from build123d import *

# Parameters (mm, degrees)
SKETCH_1_W               = 3.76
SKETCH_1_H               = 11.54
SKETCH_1_W_2             = 1.83
SKETCH_1_W_3             = 14.6
SKETCH_1_H_2             = 2.72
SKETCH_1_H_3             = 6.9
EXTRUDE_1_DEPTH          = 1
SKETCH_1_3_W             = 3.76
SKETCH_1_3_H             = 11.54
SKETCH_1_3_W_2           = 1.83
SKETCH_1_3_W_3           = 14.6
SKETCH_1_3_H_2           = 2.72
EXTRUDE_2_DEPTH          = 10
EXTRUDE_3_DEPTH          = 14.6
CUT_EXTRUDE_1_DEPTH      = 14.6
CUT_EXTRUDE_2_DEPTH      = 14.6
CUT_EXTRUDE_3_DEPTH      = 14.6
PATTERN_CIRCULAR_1_COUNT = 2
SKETCH_7_W               = 20.64829466
SKETCH_7_H               = 2.860597992
CUT_EXTRUDE_4_DEPTH      = 38.6
SKETCH_8_W               = 54.18
SKETCH_8_H               = 19.048575036
SKETCH_8_W_2             = 7
SKETCH_8_H_2             = 4.5
SKETCH_8_R               = 1.6
EXTRUDE_4_DEPTH          = 1.5
SKETCH_9_W               = 54.18
SKETCH_9_H               = 1.8
EXTRUDE_5_DEPTH          = 7
SKETCH_10_R              = 1.65
CUT_EXTRUDE_5_DEPTH      = 5
EXTRUDE_START            = 2
SKETCH_8_3_W             = 7
SKETCH_8_3_H             = 4.5
SKETCH_8_3_R             = 1.6
EXTRUDE_6_DEPTH          = 2
SKETCH_11_W              = 54.18
SKETCH_11_H              = 6.653379434
CUT_EXTRUDE_6_DEPTH      = 5
CUT_EXTRUDE_7_DEPTH      = 54.18
SKETCH_13_W              = 8.99
SKETCH_13_H              = 1
EXTRUDE_7_DEPTH          = 10


with BuildPart() as part:
    # Sketch 1 → Extrude 1 (new body)
    # profile 1 of 6: a face of its own
    with BuildSketch(Plane(origin=(0, 0, 0), x_dir=(1, 0, 0), z_dir=(0, 1, 0))):
        Polygon((-7.603, 6.17), (-7.603, -6.17), (1.387, -6.17), (1.387, -3.45), (1.387, 3.45), (1.387, 6.17), align=None)
        with Locations((-4.723, 0)):
            Rectangle(SKETCH_1_W, SKETCH_1_H, mode=Mode.SUBTRACT)
        with Locations((-0.728, 0)):
            Rectangle(SKETCH_1_W_2, SKETCH_1_H, mode=Mode.SUBTRACT)
    # profile 2 of 6: a face of its own
    with BuildSketch(Plane(origin=(0, 0, 0), x_dir=(1, 0, 0), z_dir=(0, 1, 0))):
        with Locations((8.687, -4.81)):
            Rectangle(SKETCH_1_W_3, SKETCH_1_H_2)
    # profile 3 of 6: a face of its own
    with BuildSketch(Plane(origin=(0, 0, 0), x_dir=(1, 0, 0), z_dir=(0, 1, 0))):
        with Locations((8.687, 0)):
            Rectangle(SKETCH_1_W_3, SKETCH_1_H_3)
    # profile 4 of 6: a face of its own
    with BuildSketch(Plane(origin=(0, 0, 0), x_dir=(1, 0, 0), z_dir=(0, 1, 0))):
        with Locations((8.687, 4.81)):
            Rectangle(SKETCH_1_W_3, SKETCH_1_H_2)
    # profile 5 of 6: a face of its own
    with BuildSketch(Plane(origin=(0, 0, 0), x_dir=(1, 0, 0), z_dir=(0, 1, 0))):
        with Locations((-4.723, 0)):
            Rectangle(SKETCH_1_W, SKETCH_1_H)
    # profile 6 of 6: a face of its own
    with BuildSketch(Plane(origin=(0, 0, 0), x_dir=(1, 0, 0), z_dir=(0, 1, 0))):
        with Locations((-0.728, 0)):
            Rectangle(SKETCH_1_W_2, SKETCH_1_H)
    extrude(amount=-EXTRUDE_1_DEPTH)

    # Sketch 1_3 → Extrude 2 (add)
    with BuildSketch(Plane(origin=(0, 0, 0), x_dir=(1, 0, 0), z_dir=(0, 1, 0))):
        with Locations((-4.723, 0)):
            Rectangle(SKETCH_1_3_W, SKETCH_1_3_H)
        with Locations((-0.728, 0)):
            Rectangle(SKETCH_1_3_W_2, SKETCH_1_3_H)
        with Locations((8.687, -4.81)):
            Rectangle(SKETCH_1_3_W_3, SKETCH_1_3_H_2)
        with Locations((8.687, 4.81)):
            Rectangle(SKETCH_1_3_W_3, SKETCH_1_3_H_2)
    extrude(amount=EXTRUDE_2_DEPTH)

    # Sketch 4 → Extrude 3 (add)
    with BuildSketch(Plane(origin=(15.987, 0, 0), x_dir=(0, 0, -1), z_dir=(1, 0, 0))):
        Polygon((6.17, 10), (7.707580576, 7.443577481), (7.707580576, 1.805314446), (6.17, -1), align=None)
        Polygon((-7.707580576, 1.805314446), (-6.17, -1), (-6.17, 10), (-7.707580576, 7.443577481), align=None)
    extrude(amount=-EXTRUDE_3_DEPTH)

    # Sketch 3 → Cut-Extrude 1 (cut)
    with BuildSketch(Plane(origin=(15.987, 0, 0), x_dir=(0, 0, -1), z_dir=(1, 0, 0))):
        with BuildLine():
            Line((3.45, 0), (3.743222721, 0))
            add(Edge.make_bspline(
                [(3.743222721, 0), (3.911611309, 0.15963804), (4.29393083, 0.539845441), (4.994683036, 1.333496486), (5.723480991, 2.402845903), (6.251271172, 3.695549278), (6.429364414, 5), (6.251271172, 6.304450722), (5.723480991, 7.597154097), (4.994683036, 8.666503514), (4.253106755, 9.506390689), (3.815688064, 9.935054209), (3.597380816, 10.136172737)],
                knots=[0.014828564, 0.014828564, 0.014828564, 0.014828564, 0.0625, 0.125, 0.25, 0.375, 0.5, 0.625, 0.75, 0.875, 0.9375, 0.998871937, 0.998871937, 0.998871937, 0.998871937], degree=3))
            Line((3.597380816, 10.136172737), (3.45, 10))
            Line((3.45, 10), (3.45, 0))
        make_face()
        with BuildLine():
            Line((-3.45, 0), (-3.743222721, 0))
            add(Edge.make_bspline(
                [(-3.743222721, 0), (-3.781981306, 0.035623699), (-3.849464206, 0.098316559), (-4.072000203, 0.30899054), (-4.461726475, 0.698324492), (-5.152564834, 1.48074741), (-5.881362789, 2.550096827), (-6.40915297, 3.842800202), (-6.587246212, 5.147250924), (-6.40915297, 6.451701646), (-5.881362789, 7.744405021), (-5.152564834, 8.813754438), (-4.461708764, 9.596197415), (-4.071967827, 9.985543512), (-3.84942965, 10.196217487), (-3.781968617, 10.258889811), (-3.743222721, 10.294501848)],
                knots=[0, 0, 0, 0, 0.010893382, 0.018155637, 0.0625, 0.125, 0.25, 0.375, 0.5, 0.625, 0.75, 0.875, 0.9375, 0.981850307, 0.989110184, 1, 1, 1, 1], degree=3))
            Line((-3.743222721, 10.294501848), (-3.45, 10))
            Line((-3.45, 10), (-3.45, 0))
        make_face()
    extrude(amount=-CUT_EXTRUDE_1_DEPTH, mode=Mode.SUBTRACT)

    # Sketch 5 → Cut-Extrude 2 (cut)
    with BuildSketch(Plane(origin=(0.187, 0, 0), x_dir=(0, 0, -1), z_dir=(1, 0, 0))):
        Polygon((1.17, 2.8), (-3.569711506, 4.901860767), (-5.77, 4.901860767), (-5.77, 10), (5.77, 10), (5.77, 0.3), (1.17, 0.3), align=None)
    extrude(amount=-CUT_EXTRUDE_2_DEPTH, mode=Mode.SUBTRACT)

    # Sketch 6 → Cut-Extrude 3 (cut)
    with BuildSketch(Plane(origin=(-2.843, 0, 0), x_dir=(0, 0, -1), z_dir=(1, 0, 0))):
        Polygon((1.17, 5.538552109), (1.17, 1.8), (-3.795527251, 1.8), (-5.77, 1.8), (-5.77, 5.538552109), align=None)
    extrude(amount=-CUT_EXTRUDE_3_DEPTH, mode=Mode.SUBTRACT)


with BuildPart() as pattern_circular_1_1:
    # Pattern Circular 1: pattern copy
    add(part.part.rotate(Axis((19.487, -1.5500525, 0), (0, 1, 0)), 1 * 360 / PATTERN_CIRCULAR_1_COUNT))


with BuildPart() as cut_extrude_4_tool:
    # Sketch 7 → Cut-Extrude 4 (new body)
    with BuildSketch(Plane.ZY.offset(-1.387)):
        with Locations((-0.112362095, 10.62761907)):
            Rectangle(SKETCH_7_W, SKETCH_7_H)
    extrude(amount=-CUT_EXTRUDE_4_DEPTH)


with BuildPart() as part_1:
    add(part.part)

    # Cut-Extrude 4: cut by cut_extrude_4_tool
    add(cut_extrude_4_tool.part, mode=Mode.SUBTRACT)



with BuildPart() as pattern_circular_1_1_1:
    add(pattern_circular_1_1.part)

    # Cut-Extrude 4: cut by cut_extrude_4_tool
    add(cut_extrude_4_tool.part, mode=Mode.SUBTRACT)


with BuildPart() as part_2:
    add(part_1.part)

    add(pattern_circular_1_1_1.part)  # Extrude 4 merges Pattern Circular 1_1
    # Sketch 8 → Extrude 4 (add)
    # profile 1 of 2: a face of its own
    with BuildSketch(Plane(origin=(0, 0, 0), x_dir=(1, 0, 0), z_dir=(0, 1, 0))):
        with Locations((19.487, 0)):
            Rectangle(SKETCH_8_W, SKETCH_8_H)
    # profile 2 of 2: a face of its own
    with BuildSketch(Plane(origin=(0, 0, 0), x_dir=(1, 0, 0), z_dir=(0, 1, 0))):
        with Locations((19.487, -11.774287518)):
            Rectangle(SKETCH_8_W_2, SKETCH_8_H_2)
        with Locations(Location((19.487, -11.774287518, 0), (0, 0, 270))):
            Circle(SKETCH_8_R, mode=Mode.SUBTRACT)
    extrude(amount=-EXTRUDE_4_DEPTH)

    # Sketch 9 → Extrude 5 (add)
    with BuildSketch(Plane(origin=(0, 0, 0), x_dir=(1, 0, 0), z_dir=(0, 1, 0))):
        with Locations((19.487, 8.624287518)):
            Rectangle(SKETCH_9_W, SKETCH_9_H)
    extrude(amount=EXTRUDE_5_DEPTH)

    # Sketch 10 → Cut-Extrude 5 (cut)
    with BuildSketch(Plane.XY.offset(-7.724287518)):
        with Locations((-4.603, 2.5)):
            Circle(SKETCH_10_R)
        with Locations((43.577, 2.5)):
            Circle(SKETCH_10_R)
    extrude(amount=-CUT_EXTRUDE_5_DEPTH, mode=Mode.SUBTRACT)

    # Sketch 8_3 → Extrude 6 (add)
    with BuildSketch(Plane(origin=(0, 0, 0), x_dir=(1, 0, 0), z_dir=(0, 1, 0)).offset(EXTRUDE_START)):
        with Locations((19.487, -11.774287518)):
            Rectangle(SKETCH_8_3_W, SKETCH_8_3_H)
        with Locations(Location((19.487, -11.774287518, 0), (0, 0, 270))):
            Circle(SKETCH_8_3_R, mode=Mode.SUBTRACT)
    extrude(amount=-EXTRUDE_6_DEPTH)

    # Sketch 11 → Cut-Extrude 6 (cut, symmetric)
    with BuildSketch(Plane(origin=(0, 0, 0), x_dir=(1, 0, 0), z_dir=(0, 1, 0))):
        with Locations((19.487, -11.034270293)):
            Rectangle(SKETCH_11_W, SKETCH_11_H)
    extrude(amount=CUT_EXTRUDE_6_DEPTH, both=True, mode=Mode.SUBTRACT)

    # Sketch 12 → Cut-Extrude 7 (cut)
    with BuildSketch(Plane(origin=(46.577, 0, 0), x_dir=(0, 0, -1), z_dir=(1, 0, 0))):
        Polygon((7.707580576, 1.805314446), (5.895952187, -1.5), (9.524287518, -1.5), (9.524287518, 7.146168792), (7.724287518, 7), align=None)
    extrude(amount=-CUT_EXTRUDE_7_DEPTH, mode=Mode.SUBTRACT)

    # Sketch 13 → Extrude 7 (add)
    with BuildSketch(Plane(origin=(0, 0, 0), x_dir=(1, 0, 0), z_dir=(0, 1, 0))):
        with Locations((42.082, -7.207580576)):
            Rectangle(SKETCH_13_W, SKETCH_13_H)
        with Locations((-3.108, -7.207580576)):
            Rectangle(SKETCH_13_W, SKETCH_13_H)
    extrude(amount=EXTRUDE_7_DEPTH)


solid = part_2.part
Model file for the job. Use its own axes, mm. A direction names the side the tool comes from. Give positions to 0.01 mm unless a question says otherwise; leave off trailing zeros. Loops run counter-clockwise (first coordinate to the right, second up) from the corner with the lowest first, then second, coordinate; pieces in that order, holes last.
1) Saw through at C-C (y = -0.5). Write the cut outline in (x, z), plus the area to 3 significant figures.
2) Saw through at B-B (y = 8.25). Count the separate pieces of the cut face and the enclosed holes in it, plus the area to 3 significant figures.
3) Flat gauge pins, fed straight in: pin 1 Ø2 at (y, z) = (4, 5) entering from +X; pin 2 Ø0.5 at (x, z) = (-1, -4.5) entering from +Y; pin 3 Ø2 at (y, z) = (5, -1) entering from -X; pin 4 Ø0.6 at (x, z) = (33, -6) entering from +Y. Where does each tip first touch, or does it go through?
4) Tool access for faces 4 (the flat face through (37.587, 9, 7)), 5 (the flat face through (37.587, 0.7, 7.3)), 6 (the flat face through (22.987, 5, 7)): list every direction of +Z, -Z, +X, -X, +Y, -Y with a clear straight run to the whole face (end or side of a thin tool).
5) Wall check: line 1 (X direction, y = 3.5, z = 7); line 2 (Z direction, x = 43.5, y = 0.5); line 3 (X direction, y = 0.75, z = -6.5). Give the ranges that are in metal, low to high.
6) Pull direction Z, two halves, no side cores. Call faces 1 (the flat face through (37.587, 5, -7)), 2 (the flat face through (40, 2, -5.77)), 3 (the flat face through (42, 5, 6.708)): +Z half, -Z half, draft (parallel to the pull), parting line (faces both ways), or undercut.
7) Saw through at A-A (x = 16.5). Write the cut outline in (y, z).
Answer block:
1. outline: (-7.6, -6.44) - (46.58, -6.44) - (46.58, 7.71) - (-7.6, 7.71) - close
1. area: 767 mm2
2. separate pieces: 4
2. enclosed holes: 0
2. area: 125 mm2
3. pin 1: stops at x = 0.19
3. pin 2: stops at y = 0.3
3. pin 3: passes through
3. pin 4: stops at y = 9.2
4. face 4: +Z, +Y
4. face 5: +Z
4. face 6: +Z, -Z, +Y
5. line 1: x = -7.6 to 15.99, 22.99 to 46.58
5. line 2: z = -5.77 to 1.17, 6.71 to 7.71
5. line 3: x = 1.39 to 15.99, 22.99 to 37.59
6. face 1: draft
6. face 2: -Z half
6. face 3: undercut
7. outline: (-1.5, -5.9) - (0, -6.72) - (0, 7.71) - (-1.5, 7.71) - close
